```python
from build123d import *

# Parameters (mm, degrees)
ESBO_O1_W                = 112
ESBO_O1_H                = 96
RESSALTO_EXTRUS_O1_DEPTH = 2
ESBO_O2_W                = 2
ESBO_O2_H                = 96
RESSALTO_EXTRUS_O2_DEPTH = 20
ESBO_O3_W                = 108
ESBO_O3_H                = 2
RESSALTO_EXTRUS_O3_DEPTH = 20
ESBO_O5_W                = 104
ESBO_O5_H                = 18
CORTE_EXTRUS_O1_DEPTH    = 150.1442255
ESBO_O6_R                = 3
RESSALTO_EXTRUS_O4_DEPTH = 10
ESBO_O7_R                = 1.5
CORTE_EXTRUS_O2_DEPTH    = 10
ESBO_O8_W                = 10
ESBO_O8_H                = 16
RESSALTO_EXTRUS_O5_DEPTH = 4
ESBO_O9_W                = 10
ESBO_O9_H                = 16
RESSALTO_EXTRUS_O6_DEPTH = 4
ESBO_O10_R               = 1.45
CORTE_EXTRUS_O3_DEPTH    = 150.465715132
CHANFRO2_SIZE            = 4


with BuildPart() as part:
    # Esboço1 → Ressalto-extrusão1 (new body)
    with BuildSketch(Plane(origin=(0, 0, 0), x_dir=(1, 0, 0), z_dir=(0, 1, 0))):
        with Locations((56, 48)):
            Rectangle(ESBO_O1_W, ESBO_O1_H)
    extrude(amount=RESSALTO_EXTRUS_O1_DEPTH)

    # Esboço2 → Ressalto-extrusão2 (add)
    with BuildSketch(Plane(origin=(0, 2, 0), x_dir=(1, 0, 0), z_dir=(0, 1, 0))):
        with Locations((1, 48)):
            Rectangle(ESBO_O2_W, ESBO_O2_H)
        with Locations((111, 48)):
            Rectangle(ESBO_O2_W, ESBO_O2_H)
    extrude(amount=RESSALTO_EXTRUS_O2_DEPTH)

    # Esboço3 → Ressalto-extrusão3 (add)
    with BuildSketch(Plane(origin=(0, 2, 0), x_dir=(1, 0, 0), z_dir=(0, 1, 0))):
        with Locations((56, 95)):
            Rectangle(ESBO_O3_W, ESBO_O3_H)
        with Locations((56, 1)):
            Rectangle(ESBO_O3_W, ESBO_O3_H)
        with Locations((56, 90)):
            Rectangle(ESBO_O3_W, ESBO_O3_H)
        with Locations((56, 6)):
            Rectangle(ESBO_O3_W, ESBO_O3_H)
    extrude(amount=RESSALTO_EXTRUS_O3_DEPTH)

    # Esboço5 → Corte-extrusão1 (cut, through all)
    with BuildSketch(Plane.XY):
        with Locations((56, 13)):
            Rectangle(ESBO_O5_W, ESBO_O5_H)
    extrude(amount=-CORTE_EXTRUS_O1_DEPTH, mode=Mode.SUBTRACT)

    # Esboço6 → Ressalto-extrusão4 (add)
    with BuildSketch(Plane(origin=(0, 2, 0), x_dir=(1, 0, 0), z_dir=(0, 1, 0))):
        with Locations(Location((98, 13.2, 0), (0, 0, 90))):
            Circle(ESBO_O6_R)
        with Locations(Location((14, 13.2, 0), (0, 0, 90))):
            Circle(ESBO_O6_R)
        with Locations(Location((97.143041423, 74.193980211, 0), (0, 0, 90))):
            Circle(ESBO_O6_R)
        with Locations(Location((14.151803836, 75.4, 0), (0, 0, 90))):
            Circle(ESBO_O6_R)
    extrude(amount=RESSALTO_EXTRUS_O4_DEPTH)

    # Esboço7 → Corte-extrusão2 (cut)
    with BuildSketch(Plane(origin=(0, 12, 0), x_dir=(1, 0, 0), z_dir=(0, 1, 0))):
        with Locations(Location((14.151803836, 75.4, 0), (0, 0, 270))):
            Circle(ESBO_O7_R)
        with Locations(Location((97.143041423, 74.193980211, 0), (0, 0, 270))):
            Circle(ESBO_O7_R)
        with Locations(Location((98, 13.2, 0), (0, 0, 270))):
            Circle(ESBO_O7_R)
        with Locations(Location((14, 13.2, 0), (0, 0, 270))):
            Circle(ESBO_O7_R)
    extrude(amount=-CORTE_EXTRUS_O2_DEPTH, mode=Mode.SUBTRACT)

    # Esboço8 → Ressalto-extrusão5 (add)
    with BuildSketch(Plane.ZY.offset(-110)):
        with Locations((-78, 24)):
            Rectangle(ESBO_O8_W, ESBO_O8_H)
        with Locations((-18, 24)):
            Rectangle(ESBO_O8_W, ESBO_O8_H)
    extrude(amount=RESSALTO_EXTRUS_O5_DEPTH)

    # Esboço9 → Ressalto-extrusão6 (add)
    with BuildSketch(Plane(origin=(2, 0, 0), x_dir=(0, 0, -1), z_dir=(1, 0, 0))):
        with Locations((18, 24)):
            Rectangle(ESBO_O9_W, ESBO_O9_H)
        with Locations((78, 24)):
            Rectangle(ESBO_O9_W, ESBO_O9_H)
    extrude(amount=RESSALTO_EXTRUS_O6_DEPTH)

    # Esboço10 → Corte-extrusão3 (cut, through all)
    with BuildSketch(Plane(origin=(110, 0, 0), x_dir=(0, 0, -1), z_dir=(1, 0, 0))):
        with Locations((18, 27)):
            Circle(ESBO_O10_R)
        with Locations((78, 27)):
            Circle(ESBO_O10_R)
    extrude(amount=-CORTE_EXTRUS_O3_DEPTH, mode=Mode.SUBTRACT)

    # Chanfro2
    chanfro2_edges = [part.edges().sort_by_distance(p)[0] for p in [
        (106, 16, -18),
        (106, 16, -78),
        (6, 16, -78),
        (6, 16, -18),
    ]]
    chamfer(chanfro2_edges, length=CHANFRO2_SIZE - 0.0001)  # a hair under: the kernel refuses the full size


solid = part.part
```
Verification items for the finished model (mm, model axes). A direction names the side the tool comes from. Round coordinates to 2 decimals unless told otherwise and drop trailing zeros. Write each loop counter-clockwise with the first axis right and the second up, starting at its lowest first coordinate (ties: lowest second). Pieces come first, ordered by that corner, then holes.
1. Draft check along Z on faces 4 (the flat face through (106, 25, -78)), 5 (the flat face through (108, 26, -13)), 6 (the flat face through (56, 3, -96)). Enter one of: +Z half, -Z half, draft (parallel to the pull), parting line (faces both ways), or undercut.
2. Access from +Z, -Z, +X, -X, +Y, -Y to the whole of each face (thin tool, end or side, straight path). Record for faces 1 (the flat face through (106, 25, -18)), 2 (the flat face through (108, 18, -78)), 3 (the cylindrical face through (16.662, 6.93, -14.584)).
3. Section check A-A on z = -18. State how many separate pieces and enclosed holes the cut face has, plus the area to 3 significant figures.
4. Gauge pin test, flat ends, axial feed: P1, Ø8, axis at x = 14.5, z = -74, coming from the +Y side; P2, Ø2, axis at y = 11, z = -1, coming from the -X side; P3, Ø5, axis at x = 97.5, y = 12.5, coming from the -Z side; P4, Ø2, axis at x = 1.5, z = -37.5, coming from the +Y side. Record the tip position at first contact, or that the pin passes through.
5. Section check C-C on z = -62. Enter the section's corners in (x, y), plus the area to 3 significant figures.
6. Scan lines: L1, parallel to X at y = 9.5, z = -13.2; L2, parallel to X at y = 12, z = -70.5; L3, parallel to X at y = 20, z = -15. Record each from-to range of solid material in increasing order.
7. Section check D-D on x = 26.5. Enter the section's corners in (y, z).
Answer:
1. face 4: draft
1. face 5: undercut
1. face 6: -Z half
2. face 1: +Z, -Z, +Y
2. face 2: none
2. face 3: +Y
3. separate pieces: 3
3. enclosed holes: 0
3. area: 393 mm2
4. P1: stops at y = 12
4. P2: stops at x = 0
4. P3: stops at z = -77.19
4. P4: stops at y = 22
5. outline: (0, 0) - (112, 0) - (112, 22) - (110, 22) - (110, 2) - (2, 2) - (2, 22) - (0, 22) - close
5. area: 304 mm2
6. L1: x = 0 to 2, 11 to 12.5, 15.5 to 17, 95 to 96.5, 99.5 to 101, 110 to 112
6. L2: x = 0 to 2, 110 to 112
6. L3: x = 0 to 6, 106 to 112
7. outline: (0, -96) - (4, -96) - (4, -94) - (2, -94) - (2, -91) - (4, -91) - (4, -89) - (2, -89) - (2, -7) - (4, -7) - (4, -5) - (2, -5) - (2, -2) - (4, -2) - (4, 0) - (0, 0) - close
